Can you work these out from the drawing? Everything is in mm from the part's minimum corner. Round coordinates to 2 decimals unless told otherwise and drop trailing zeros. Loops run counter-clockwise (first coordinate to the right, second up) from the corner with the lowest first, then second, coordinate; pieces in that order, holes last. Notation, with made-up numbers: (-36, 49.5) - (-9, 49.5) arc R27 ccw to (-9, 87.5) - close; hole circle Ø9 at (3.5, -18). An arc over 180 degrees is marked (long way). Answer as a JSON object with one key per item and string values. Group by question number.
1) I want a section at C-C, the plane z = 135. Please give me the cut outline in (x, y).
2) Will this pin go through, and if not, where does the flat tip stop? P1, Ø1.9, axis at y = 3.5, z = 135.5, coming from the -X side.
3) I want a section at B-B, the plane y = 3. Please give me the cut outline in (x, z).
4) If I drill on line 1 along Z through (x, y) = (25.4, 2); line 2 along X through (y, z) = (3.75, 254); line 3 along Z through (x, y) = (50.5, 5.25), over which ranges is the centre line in solid material (lowest first)? Write a range as [from, to].
5) I want a section at A-A, the plane x = 37. Please give me the cut outline in (y, z).
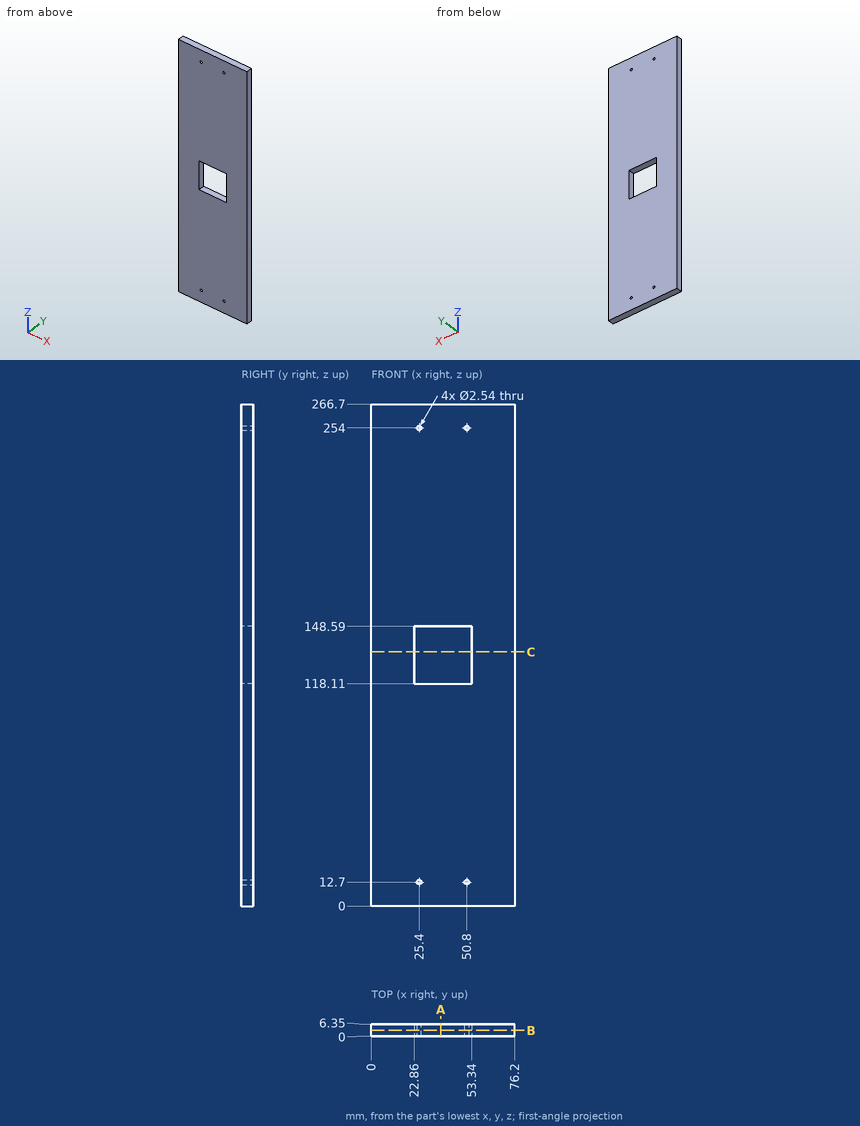
Outcome:
{
 "1": {"outline": "(0, 0) - (22.86, 0) - (22.86, 6.35) - (0, 6.35) - close; (53.34, 0) - (76.2, 0) - (76.2, 6.35) - (53.34, 6.35) - close"},
 "2": {"P1": "x = 0"},
 "3": {"outline": "(0, 0) - (76.2, 0) - (76.2, 266.7) - (0, 266.7) - close; hole (22.86, 118.11) - (53.34, 118.11) - (53.34, 148.59) - (22.86, 148.59) - close; hole circle Ø2.54 at (25.4, 12.7); hole circle Ø2.54 at (25.4, 254); hole circle Ø2.54 at (50.8, 12.7); hole circle Ø2.54 at (50.8, 254)"},
 "4": {"line 1": "[0, 11.43], [13.97, 118.11], [148.59, 252.73], [255.27, 266.7]", "line 2": "[0, 24.13], [26.67, 49.53], [52.07, 76.2]", "line 3": "[0, 11.47], [13.93, 118.11], [148.59, 252.77], [255.23, 266.7]"},
 "5": {"outline": "(0, 0) - (6.35, 0) - (6.35, 118.11) - (0, 118.11) - close; (0, 148.59) - (6.35, 148.59) - (6.35, 266.7) - (0, 266.7) - close"}
}
